Autodesk Inventor part; units mm, degrees
ref_plane "YZ Plane" through (0, 0, 0) normal (1, 0, 0) x (0, 1, 0)
ref_plane "XZ Plane" through (0, 0, 0) normal (0, 1, 0) x (-1, 0, 0)
ref_plane "XY Plane" through (0, 0, 0) normal (0, 0, 1) x (1, 0, 0)
sketch "Sketch1" plane through (0, 0, 0) normal (0, 1, 0) x (-1, 0, 0)
  line L0 (0, 31.75) -> (-3.175, 31.75)
  line L1 (-3.175, -31.75) -> (0, -31.75)
  line L2 (0, -31.75) -> (0, 31.75)
  circle A0 centre (-18.85, 0) radius 12.5
  circle A1 centre (-18.85, 0) radius 12.2
  arc A2 (-18.85, 15.675) -> (-18.85, -15.675) centre (-18.85, 0) ccw
  line L3 (-18.85, 15.675) -> (-6.35, 15.675)
  line L4 (-18.85, -15.675) -> (-6.35, -15.675)
  line L5 (-3.175, 31.75) -> (-3.175, 18.85)
  line L6 (-3.175, -18.85) -> (-3.175, -31.75)
  arc A3 (-6.35, 15.675) -> (-3.175, 18.85) centre (-6.35, 18.85) ccw
  arc A4 (-3.175, -18.85) -> (-6.35, -15.675) centre (-6.35, -18.85) ccw
  point P0 (0, 0)
  dimension "d0" = 3.175
  dimension "d1" = 63.5
  dimension "d4" = 25
  dimension "d6" = 24.4
  dimension "d7" = 31.35
  dimension "d8" = 3.175
  dimension "d26" = 3.175
  dimension "d27" = 18.85
extrude "Extrusion1" add sketch "Sketch1" along normal blind 49.8 contours L2 L1 L6 A4 L4 A2 L3 A3 L5 L0
extrude "Extrusion2" add sketch "Sketch1" along normal blind 30.8 contours A0
sketch "Sketch2" plane through (3.175, 0, 31.75) normal (1, 0, 0) x (0, 0, -1)
  line L0 (63.5, 0) -> (63.5, 49.8)
  line L1 (0, 0) -> (0, 49.8)
  circle A0 centre (6.35, 28.6333) radius 1.5875
  circle A1 centre (6.35, 7.4667) radius 1.5875
  line L2 (0, 49.8) -> (12.9, 49.8)
  line L3 (31.75, 0) -> (31.75, 49.8)
  line L4 (19.25, 49.8) -> (44.25, 49.8)
  circle A2 centre (57.15, 28.6333) radius 1.5875
  circle A3 centre (57.15, 7.4667) radius 1.5875
  dimension "d14" = 63.5
  dimension "d16" = 3.175
  dimension "d17" = 3.175
  dimension "d18" = 21.1667
  dimension "d19" = 21.1667
  dimension "d20" = 0
  dimension "d21" = 6.35
  dimension "d22" = 31.75
extrude "Extrusion3" cut sketch "Sketch2" against normal blind 3.175
properties part number "Motor_Mount_3DPrint"
Can you work these out from the model? Positions are in its coordinate system, mm. A direction names the side the tool comes from. Round coordinates to 2 decimals unless told otherwise and drop trailing zeros. Loops run counter-clockwise (first coordinate to the right, second up) from the corner with the lowest first, then second, coordinate; pieces in that order, holes last. Notation, with made-up numbers: (57, 73.5) - (64, 73.5) arc R16 ccw to (64, 86.5) - close; hole circle Ø4 at (-35, 45). An arc over 180 degrees is marked (long way). Write item = value, one per line. Start each with the question number.
(1) If we section it at C-C (z = -25.4): Please give me the cut outline in (x, y) (3 decimals), and give its area (3 significant figures).
(2) If we mould it in two halves opening along X, with no side actions, what happens to faces 4 (the face through (2, 25, 31.75)), 5 (the face through (4.08, 24.55, 16.63)), 6 (the face through (31.04, 15.18, -0.54))? For each: released by +X, released by -X, zero draft, split by the parting line, or undercut.
(3) If we section it at D-D (x = 11.5): Please give me the cut outline in (y, z) (3 decimals).
(4) For faces 1 (the face through (3.175, 25, 25)), 2 (the face through (6.927, 40.167, -3.755)), 3 (the face through (13, 25, -15.675)), which set-ups out of +Z, -Z, +X, -X, +Y, -Y let a thin tool reach every point of the face, with its end or its side?
(5) If we section it at B-B (y = 39): Please give me the cut outline in (x, z) (3 decimals), and give its area (3 significant figures).
(6) If we section it at A-A (z = 0): Please give me the cut outline in (x, y) (3 decimals).
(7) For P1, Ø4, axis at x = 15.5, y = 34.5, coming from the -Z side (3 decimals); P2, Ø5, axis at y = 42.5, z = -24.5, coming from the +X side (3 decimals); P3, Ø3, axis at y = 10.5, z = -12.5, coming from the +X side; P4, Ø15, axis at x = 18.85, z = 0, coming from the -Y side, each with a flat end and sliding along its axis, tell me the tip position at first contact or that it passes through.
(8) If I drill on probe 1 along Y at (x, z) = (2.2, 25.4); probe 2 along Z at (x, y) = (18.85, 38) (3 decimals); probe 3 along X at (y, z) = (41, -28.5) (3 decimals), over which ranges is the centre line in solid material (lowest first)? Write a range as [from, to].
Ans:
q1.outline = (0, 0) - (3.175, 0) - (3.175, 5.879) - (0, 5.879) - close; (0, 9.054) - (3.175, 9.054) - (3.175, 27.046) - (0, 27.046) - close; (0, 30.221) - (3.175, 30.221) - (3.175, 49.8) - (0, 49.8) - close
q1.area = 138 mm²
q2.face_4 = zero draft
q2.face_5 = released by +X
q2.face_6 = undercut
q3.outline = (0, -15.675) - (49.8, -15.675) - (49.8, -10.111) - (30.8, -10.111) - (30.8, -9.737) - (0, -9.737) - close; (0, 9.737) - (30.8, 9.737) - (30.8, 10.111) - (49.8, 10.111) - (49.8, 15.675) - (0, 15.675) - close
q4.face_1 = +Z, +X, +Y, -Y
q4.face_2 = +Y
q4.face_3 = -Z, +X, +Y, -Y
q5.outline = (0, -31.75) - (3.175, -31.75) - (3.175, -18.85) arc R3.175 cw to (6.35, -15.675) - (18.85, -15.675) arc R15.675 ccw to (18.85, 15.675) - (6.35, 15.675) arc R3.175 cw to (3.175, 18.85) - (3.175, 31.75) - (0, 31.75) - close; hole circle Ø25 at (18.85, 0)
q5.area = 592 mm²
q6.outline = (0, 0) - (6.65, 0) - (6.65, 30.8) - (6.35, 30.8) - (6.35, 49.8) - (0, 49.8) - close; (31.05, 0) - (34.525, 0) - (34.525, 49.8) - (31.35, 49.8) - (31.35, 30.8) - (31.05, 30.8) - close
q7.P1 = -15.675
q7.P2 = 3.175
q7.P3 = 30.02
q7.P4 = through
q8.probe_1 = [0, 5.88], [9.05, 27.05], [30.22, 49.8]
q8.probe_2 = [-15.675, -12.5], [12.5, 15.675]
q8.probe_3 = [0, 3.175]
